Here's how the part is built. I have some questions about the finished solid (model axes, mm). Round coordinates to 2 decimals unless told otherwise and drop trailing zeros. One line per item, written item: value.
from build123d import *

# Parameters (mm, degrees)
SKETCH8_R          = 142.345864783
CUT_EXTRUDE4_DEPTH = 524.976683945
SKETCH9_R          = 2.286
CUT_EXTRUDE5_DEPTH = 10.16


# Read off the part's stored shape, not the designer's step: Revolve1
with BuildPart() as part:
    # Revolve1 outline → Revolve1 (revolve)
    with BuildSketch(Plane(origin=(0, -76.2, 0), x_dir=(0, 1, 0), z_dir=(0, 0, -1))):
        with BuildLine():
            Line((87.660570284, -259.812483715), (87.660570284, 6.35))
            Line((87.660570284, 6.35), (76.2, 6.35))
            Line((76.2, 6.35), (76.2, 0))
            add(Edge.make_bspline(
                [(76.2, 0), (76.2, -50.8), (76.2, -101.6), (76.2, -157.182375328), (76.2, -166.747125983), (76.2, -181.094251966), (76.2, -190.659002621), (76.2, -199.585120865), (76.2, -207.872606698), (76.045040161, -220.304800851), (75.838475179, -228.589711976), (75.676289458, -235.094659099), (75.558482998, -239.819642219), (75.408519742, -245.046645359), (75.323959024, -247.911294959), (75.309046779, -248.413737762)],
                knots=[0.761574077, 0.761574077, 0.761574077, 0.761574077, 0.907841521, 0.907841521, 0.921611321, 0.935381121, 0.94915092, 0.94915092, 0.961081918, 0.973012916, 0.984943914, 0.984943914, 0.991748303, 0.998552693, 1, 1, 1, 1], degree=3))
            ThreePointArc((75.309046779, -248.413737762), (76.063072477, -251.60858665), (78.31179575, -254))
            ThreePointArc((78.31179575, -254), (80.564993874, -256.399753184), (81.313954963, -259.605182082))
            add(Edge.make_bspline(
                [(81.313954963, -259.605182082), (81.068244998, -267.127682546), (80.485669281, -283.426031509), (79.080505646, -317.270262329), (76.911244662, -361.130016616), (72.828043506, -431.275457269), (67.933123727, -501.372917975), (62.308317352, -571.414486843), (57.722301111, -623.914744737), (52.760650205, -676.380314027), (47.400937928, -728.80566324), (42.572514827, -772.453634614), (38.460845457, -807.34181653), (35.241099853, -833.490683911), (31.871058885, -859.619375692), (28.330664868, -885.723877265), (25.622093078, -904.612492975), (24.105535605, -914.800968172), (23.880348875, -916.305282206)],
                knots=[0.121539178, 0.121539178, 0.121539178, 0.121539178, 0.143122913, 0.168303261, 0.218663957, 0.269024652, 0.369746043, 0.420106738, 0.470467434, 0.520828129, 0.571188825, 0.62154952, 0.646729868, 0.671910216, 0.697090564, 0.722270911, 0.747451259, 0.75181382, 0.75181382, 0.75181382, 0.75181382], degree=3))
            ThreePointArc((23.880348875, -916.305282206), (21.744774169, -920.17623014), (17.600321371, -921.7152))
            Line((17.600321371, -921.7152), (17.600321371, -928.0652))
            ThreePointArc((17.600321371, -928.0652), (25.889226967, -924.987260279), (30.160376378, -917.245364413))
            add(Edge.make_bspline(
                [(30.160376378, -917.245364413), (34.234797238, -890.027026607), (41.61127386, -835.465785428), (54.429099246, -726.176632388), (67.687881192, -589.280273052), (78.033524736, -452.140135716), (84.371569009, -342.298022137), (86.762340852, -287.31210638), (87.660570284, -259.812483715)],
                knots=[0.750906811, 0.750906811, 0.750906811, 0.750906811, 0.829691141, 0.908475472, 1.066044132, 1.223612793, 1.302397123, 1.381181453, 1.381181453, 1.381181453, 1.381181453], degree=3))
        make_face()
    revolve(axis=Axis((0, -76.2, 0), (1, 0, 0)))

    # Sketch8 → Cut-Extrude4 (cut, through all)
    with BuildSketch(Plane(origin=(-438.15, 0, 0), x_dir=(0, 0, -1), z_dir=(1, 0, 0))):
        with Locations((0, -76.2)):
            Circle(SKETCH8_R)
    extrude(amount=CUT_EXTRUDE4_DEPTH, mode=Mode.SUBTRACT)

    # Sketch9 → Cut-Extrude5 (cut)
    with BuildSketch(Plane(origin=(-438.15, 0, 0), x_dir=(0, 0, -1), z_dir=(1, 0, 0))):
        with Locations((23.926020811, -4.692661383)):
            Circle(SKETCH9_R)
        with Locations((61.387516514, -32.412710015)):
            Circle(SKETCH9_R)
        with Locations((75.401067393, -76.858015146)):
            Circle(SKETCH9_R)
        with Locations((60.613973316, -121.051980857)):
            Circle(SKETCH9_R)
        with Locations((22.674401626, -148.114014343)):
            Circle(SKETCH9_R)
        with Locations((-23.926020811, -147.707338617)):
            Circle(SKETCH9_R)
        with Locations((-61.387516514, -119.987289985)):
            Circle(SKETCH9_R)
        with Locations((-75.401067393, -75.541984854)):
            Circle(SKETCH9_R)
        with Locations((-60.613973316, -31.348019143)):
            Circle(SKETCH9_R)
        with Locations((-22.674401626, -4.285985657)):
            Circle(SKETCH9_R)
    extrude(amount=-CUT_EXTRUDE5_DEPTH, mode=Mode.SUBTRACT)


solid = part.part
Q1. We'd pull the mould along Y, two halves only. Please class faces 1 (the flat face through (-438.15, -140, -35)), 2 (the cylindrical face through (-924.935, -59.412, 5.287)): released by +Y, released by -Y, zero draft, split by the parting line, or undercut.
Results list:
face 1: zero draft
face 2: undercut
Q2. If I drill on line 1 along Z through (x, y) = (-506, -30.5); line 2 along Z through (x, y) = (-660, -44); line 3 along Y through (x, z) = (-681.5, 21), over which ranges is the centre line in solid material (lowest first)?
Results list:
line 1: -57.97 to -49.6, 49.6 to 57.97
line 2: -51.42 to -43.71, 43.71 to 51.42
line 3: -130.88 to -123.98, -28.42 to -21.52
Q3. Will these pins go through, and if not, where does the flat tip stop? pin 1 (5.5 mm diameter, centred on y = -76.86, z = -75.4, fed in from +X); pin 2 (1.4 mm diameter, centred on y = -148, z = -23, fed in from +X); pin 3 (5 mm diameter, centred on x = -632, z = -48, fed in from +Y); pin 4 (4 mm diameter, centred on x = -865.5, y = -39.5, fed in from -Z).
Results list:
pin 1: x = -438.15
pin 2: x = -448.31
pin 3: y = -32.17
pin 4: z = -14.19
